Geometry: final body of the model. Coordinates: model frame, mm. A direction names the side the tool comes from. Give positions to 0.01 mm unless a question says otherwise; leave off trailing zeros.
1. First-contact query: P1, Ø1.5, axis at x = 24.5, z = 13, coming from the -Y side; P2, Ø1.5, axis at x = 5.5, y = 16, coming from the +Z side; P3, Ø2, axis at x = -97, y = 10, coming from the +Z side. Flat tips, straight axial feed; report the tip coordinate or a pass-through.
2. Material intervals for line 1 along X through (y, z) = (7, 19.5); line 2 along X through (y, z) = (14, 24); line 3 along Z through (x, y) = (-47.5, 20), sorted ascending.
3. Access query for faces 1 (the face through (20, 17, 75.018)), 2 (the face through (-93.177, 15, 32)). Directions: +Z, -Z, +X, -X, +Y, -Y. A direction counts if a zero-diameter tool reaches every point of the face in a straight line with its end or side. Return the directions, or none.
4. Draft query along X for faces 3 (the face through (20.213, 16.035, 18.911)), 4 (the face through (-96, 14, -54.482)). Return one class per face: +X half, -X half, draft (parallel to the pull), parting line (faces both ways), or undercut.
from build123d import *

# Parameters (mm, degrees)
SKETCH1_W           = 240
SKETCH1_H           = 351.15
BOSS_EXTRUDE3_DEPTH = 21
SKETCH5_W           = 248.975913499
SKETCH5_H           = 113.170869772
CUT_EXTRUDE5_DEPTH  = 254
CAVITY1_START       = -93.176553254
CAVITY1_DEPTH       = 230
SKETCH6_W           = 230
SKETCH6_H           = 2.384694545
CUT_EXTRUDE6_DEPTH  = 10
SKETCH7_W           = 329.692379319
SKETCH7_H           = 158.801284786
CUT_EXTRUDE10_DEPTH = 41
SKETCH11_W          = 230
SKETCH11_H          = 3.476591165
CUT_EXTRUDE14_DEPTH = 10
SKETCH9_W           = 2.6
SKETCH9_H           = 130.2
BOSS_EXTRUDE4_DEPTH = 12
SKETCH14_R          = 2.021585834
CUT_EXTRUDE15_DEPTH = 10
CUT_EXTRUDE16_START = -10
SKETCH13_R          = 2.021585834
CUT_EXTRUDE16_DEPTH = 10
SKETCH16_R          = 2
CUT_EXTRUDE17_DEPTH = 10
CUT_EXTRUDE18_START = -10
SKETCH15_R          = 2
CUT_EXTRUDE18_DEPTH = 10


with BuildPart() as part:
    # Sketch1 → Boss-Extrude3 (new body)
    with BuildSketch(Plane(origin=(0, 0, 0), x_dir=(1, 0, 0), z_dir=(0, 1, 0))):
        with Locations((21.823446746, 98.176553254)):
            Rectangle(SKETCH1_W, SKETCH1_H)
    extrude(amount=BOSS_EXTRUDE3_DEPTH)

    # Sketch5 → Cut-Extrude5 (cut)
    with BuildSketch(Plane(origin=(0, 0, -54.481553254), x_dir=(-1, 0, 0), z_dir=(0, 0, -1))):
        with Locations((-20.8478358, 4.110963623)):
            Rectangle(SKETCH5_W, SKETCH5_H)
    extrude(amount=CUT_EXTRUDE5_DEPTH, mode=Mode.SUBTRACT)

    # Cavity1: read off the stored shape, not the designer's step
    # Cavity1 outline → Cavity1 (cut)
    with BuildSketch(Plane.YZ.offset(CAVITY1_START)):
        Polygon((18.5, 60.403141291), (13.5, 67.518446746), (13.5, 67.903141291), (18.5, 67.903141291), (13.5, 75.018446746), (5, 75.018446746), (5, -54.481553254), (13.5, -54.481553254), (13.5, -52.096858709), (18.5, -52.096858709), (13.5, -44.981553254), (13.5, -44.596858709), (18.5, -44.596858709), (13.5, -37.481553254), (13.5, -37.096858709), (18.5, -37.096858709), (13.5, -29.981553254), (13.5, -29.596858709), (18.5, -29.596858709), (13.5, -22.481553254), (13.5, -22.096858709), (18.5, -22.096858709), (13.5, -14.981553254), (13.5, -14.596858709), (18.5, -14.596858709), (13.5, -7.481553254), (13.5, -7.096858709), (18.5, -7.096858709), (13.5, 0.018446746), (13.5, 0.403141291), (18.5, 0.403141291), (13.5, 7.518446746), (13.5, 7.903141291), (18.5, 7.903141291), (13.5, 15.018446746), (13.5, 15.403141291), (18.5, 15.403141291), (13.5, 22.518446746), (13.5, 22.903141291), (18.5, 22.903141291), (13.5, 30.018446746), (13.5, 30.403141291), (18.5, 30.403141291), (13.5, 37.518446746), (13.5, 37.903141291), (18.5, 37.903141291), (13.5, 45.018446746), (13.5, 45.403141291), (18.5, 45.403141291), (13.5, 52.518446746), (13.5, 52.903141291), (18.5, 52.903141291), (13.5, 60.018446746), (13.5, 60.403141291), align=None)
    extrude(amount=CAVITY1_DEPTH, mode=Mode.SUBTRACT)

    # Sketch6 → Cut-Extrude6 (cut)
    with BuildSketch(Plane(origin=(0, 13.5, 0), x_dir=(-1, 0, 0), z_dir=(0, -1, 0))):
        with Locations((-21.823446746, 53.289205982)):
            Rectangle(SKETCH6_W, SKETCH6_H)
    extrude(amount=-CUT_EXTRUDE6_DEPTH, mode=Mode.SUBTRACT)

    # Sketch7 → Cut-Extrude10 (cut)
    with BuildSketch(Plane(origin=(0, 13.5, 0), x_dir=(-1, 0, 0), z_dir=(0, -1, 0))):
        with Locations((-33.84938791, -12.885366014)):
            Rectangle(SKETCH7_W, SKETCH7_H)
    extrude(amount=CUT_EXTRUDE10_DEPTH, mode=Mode.SUBTRACT)

    # Sketch11 → Cut-Extrude14 (cut)
    with BuildSketch(Plane.XZ.offset(-13.5)):
        with Locations((21.823446746, 76.756742329)):
            Rectangle(SKETCH11_W, SKETCH11_H)
    extrude(amount=-CUT_EXTRUDE14_DEPTH, mode=Mode.SUBTRACT)

    # Sketch9 → Boss-Extrude4 (add)
    with BuildSketch(Plane.XZ.offset(-13.5)):
        with Locations((-96.876553254, 10.618446746)):
            Rectangle(SKETCH9_W, SKETCH9_H)
        with Locations((140.523446746, 10.618446746)):
            Rectangle(SKETCH9_W, SKETCH9_H)
    extrude(amount=BOSS_EXTRUDE4_DEPTH)

    # Sketch14 → Cut-Extrude15 (cut)
    with BuildSketch(Plane.ZY.offset(98.176553254)):
        with Locations((11.458446746, 4.5)):
            Circle(SKETCH14_R)
    extrude(amount=-CUT_EXTRUDE15_DEPTH, mode=Mode.SUBTRACT)

    # Sketch13 → Cut-Extrude16 (cut)
    with BuildSketch(Plane(origin=(141.823446746, 0, 0), x_dir=(0, 0, -1), z_dir=(1, 0, 0)).offset(CUT_EXTRUDE16_START)):
        with Locations(Location((-11.458446746, 4.5, 0), (0, 0, 180))):
            Circle(SKETCH13_R)
    extrude(amount=CUT_EXTRUDE16_DEPTH, mode=Mode.SUBTRACT)

    # Sketch16 → Cut-Extrude17 (cut)
    with BuildSketch(Plane(origin=(141.823446746, 0, 0), x_dir=(0, 0, -1), z_dir=(1, 0, 0))):
        with Locations((-61.32678821, 4.5)):
            Circle(SKETCH16_R)
    extrude(amount=-CUT_EXTRUDE17_DEPTH, mode=Mode.SUBTRACT)

    # Sketch15 → Cut-Extrude18 (cut)
    with BuildSketch(Plane.ZY.offset(98.176553254).offset(CUT_EXTRUDE18_START)):
        with Locations(Location((61.32678821, 4.5, 0), (0, 0, 180))):
            Circle(SKETCH15_R)
    extrude(amount=CUT_EXTRUDE18_DEPTH, mode=Mode.SUBTRACT)


solid = part.part
Answers below:
1. P1: stops at y = 14.39
1. P2: stops at z = 75.02
1. P3: stops at z = 75.72
2. line 1: x = -98.18 to -95.58, 139.22 to 141.82
2. line 2: x = -98.18 to -93.18, 136.82 to 141.82
2. line 3: z = -52.1 to 75.02
3. face 1: +Z, +Y, -Y
3. face 2: -Y
4. face 3: undercut
4. face 4: draft
